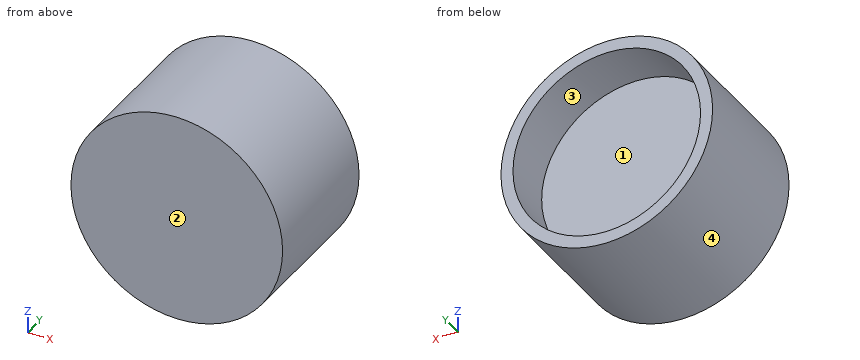
Autodesk Fusion 360 part; units mm, degrees
sketch "Sketch1" plane through (0, 0, 0) normal (0, 0, 1) x (1, 0, 0)
  curve L0
  curve L1
  curve L2
  curve L3
sketch "Sketch2" plane through (0, 0, 0) normal (0, 1, 0) x (1, 0, 0)
  circle A0 centre (-0.0361, -7.2532) radius 6.2056
extrude "Extrude2" add sketch "Sketch2" along normal blind 11
hole "Hole1" at (-1.2862, 11, 9.8296) direction (0, -1, 0) diameter 19 depth 3 tip angle 180
hole "Hole2" at (-0.0361, 8, 7.2532) direction (0, -1, 0) diameter 11 depth 3 tip angle 180
Source: CAD feature listing. Evaluate the final solid. Frame: model axes, mm. Face numbers are marked on the shaded views. Round coordinates to 2 decimals unless told otherwise and drop trailing zeros. Loops run counter-clockwise (first coordinate to the right, second up) from the corner with the lowest first, then second, coordinate; pieces in that order, holes last. Notation, with made-up numbers: (-3.75, 59.5) - (12.25, 59.5) arc R19 ccw to (12.25, 73.5) - close; hole circle Ø2 at (69, -36.5). An arc over 180 degrees is marked (long way). Write item = value, one per line. Start each with the question number.
Item 1: Material intervals for line 1 (Y direction, x = 3.5, z = 10.5); line 2 (Z direction, x = 0.25, y = 6.25); line 3 (Z direction, x = 4, y = 5.25), sorted ascending.
Item 2: Section query C-C on y = 1. Output: boundary loops of the cut face in (x, z).
Item 3: Section query D-D on y = 5.25. Output: boundary loops of the cut face in (x, z).
Item 4: First-contact query: pin 1 Ø3 at (x, y) = (4, 1) entering from -Z; pin 2 Ø6.5 at (x, z) = (-0.04, 7.25) entering from +Y; pin 3 Ø2 at (y, z) = (4.5, 10.5) entering from +X. Flat tips, straight axial feed; report the tip coordinate or a pass-through.
Item 5: Section query A-A on x = -3.5. Output: boundary loops of the cut face in (y, z), plus the area to 3 significant figures.
Item 6: Mould query, pull axis X, two halves, no side actions, for the marked faces 1, 2, 3 and 4. Classes: released by +X, released by -X, zero draft, split by the parting line, or undercut.
Item 7: Section query B-B on z = 2.25. Output: boundary loops of the cut face in (x, y).
Results list:
q1.line_1 = 0 to 5
q1.line_2 = 1.05 to 1.76, 12.75 to 13.45
q1.line_3 = 2.54 to 3.52, 10.99 to 11.97
q2.outline = circle Ø12.41 at (-0.04, 7.25)
q3.outline = circle Ø12.41 at (-0.04, 7.25); hole circle Ø11 at (-0.04, 7.25)
q4.pin_1 = 1.59
q4.pin_2 = 5
q4.pin_3 = 5.75
q5.outline = (0, 2.1) - (8, 2.1) - (8, 2.98) - (5, 2.98) - (5, 11.53) - (8, 11.53) - (8, 12.4) - (0, 12.4) - close
q5.area = 56.7 mm²
q6.face_1 = undercut
q6.face_2 = zero draft
q6.face_3 = undercut
q6.face_4 = split by the parting line
q7.outline = (-3.71, 0) - (3.64, 0) - (3.64, 8) - (2.25, 8) - (2.25, 5) - (-2.32, 5) - (-2.32, 8) - (-3.71, 8) - close
